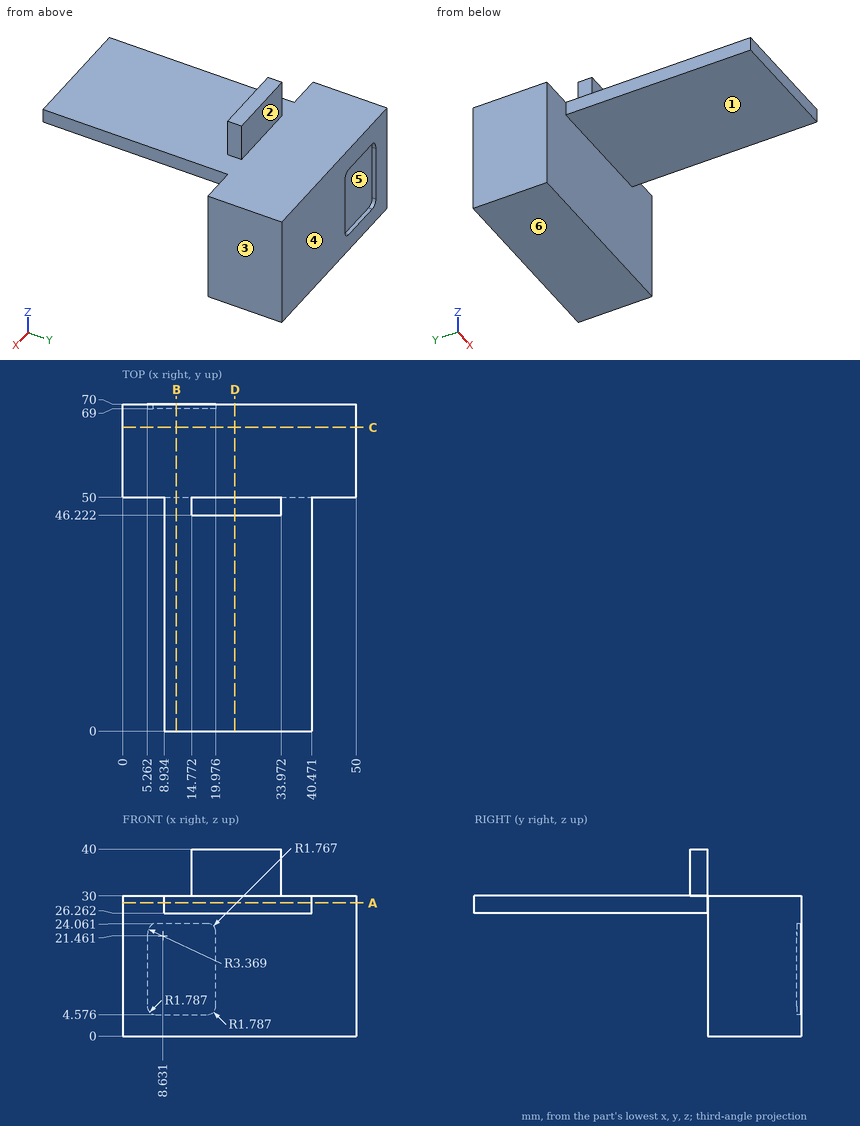
Drawing for the job (mm, zero at the part's lowest x, y, z). A direction names the side the tool comes from. Give positions to 0.01 mm unless a question says otherwise; leave off trailing zeros. Loops run counter-clockwise (first coordinate to the right, second up) from the corner with the lowest first, then second, coordinate; pieces in that order, holes last.
(1) Band-saw the part on A-A (z = 28.5). Write the cut outline in (x, y), and give its area (3 significant figures).
Return value:
outline: (0, 50) - (8.93, 50) - (8.93, 0) - (40.47, 0) - (40.47, 50) - (50, 50) - (50, 70) - (0, 70) - close
area: 2,580 mm2
(2) Pull direction Z, two halves, no side cores. Call the marked faces 4, 5 and 6: pulls with the +Z half, pulls with the -Z half, needs draft (parallel to the pull), parting line crosses it, or undercut.
Return value:
face 4: needs draft
face 5: undercut
face 6: pulls with the -Z half
(3) 3-axis set-ups, long thin cutter, end or side, ignore diameter. For the marked faces 1, 2 and 3: which of +Z, -Z, +X, -X, +Y, -Y reach the whole face in a straight line?
Return value:
face 1: -Z, +X, -X, -Y
face 2: +Z, +X, -X, +Y
face 3: +Z, -Z, +X, +Y, -Y
(4) Band-saw the part on B-B (x = 11.5). Write the cut outline in (y, z) (1 decimal).
Return value:
outline: (0, 26.3) - (50, 26.3) - (50, 0) - (70, 0) - (70, 4.6) - (69, 4.6) - (69, 24.1) - (70, 24.1) - (70, 30) - (0, 30) - close
(5) Drill centre lines: line 1 along X through (y, z) = (21, 27); line 2 along Z through (x, y) = (10.5, 19); line 3 along Y through (x, z) = (35, 18.5). Where is each one in solid material? Low to high.
Return value:
line 1: x = 8.93 to 40.47
line 2: z = 26.26 to 30
line 3: y = 50 to 70
(6) Pin check, flat tips, straight feed: pin 1 (3 mm diameter, centred on x = 19, y = 44, fed in from -Z); pin 2 (3 mm diameter, centred on x = 21.5, z = 37.5, fed in from -Y); pin 3 (3 mm diameter, centred on y = 48.5, z = 35, fed in from -X). Stop position of each tip, or through.
Return value:
pin 1: stops at z = 26.26
pin 2: stops at y = 46.22
pin 3: stops at x = 14.77
(7) Band-saw the part on D-D (x = 24). Write the cut outline in (y, z).
Return value:
outline: (0, 26.26) - (50, 26.26) - (50, 0) - (70, 0) - (70, 30) - (50, 30) - (50, 40) - (46.22, 40) - (46.22, 30) - (0, 30) - close
(8) Band-saw the part on C-C (y = 65). Write the cut outline in (x, z).
Return value:
outline: (0, 0) - (50, 0) - (50, 30) - (0, 30) - close
